Input: part model. Units: mm. Frame: model coordinates. A direction names the side the tool comes from. Coordinates: 2 decimals unless noted, no trailing zeros. Loops run counter-clockwise (first coordinate to the right, second up) from the corner with the lowest first, then second, coordinate; pieces in that order, holes last. Notation, with made-up numbers: (59.25, 34.5) -> (110.25, 34.5) arc R18 cw to (110.25, 43.5) -> close; hole circle Ø9 at (-7, 37). An arc over 180 degrees is marked (long way). Answer as a JSON object with one key per item and string values.
from build123d import *

# Parameters (mm, degrees)
SKETCH1_W            = 42
SKETCH1_H            = 84
SKETCH1_R            = 11.5
BOSS_EXTRUDE1_DEPTH  = 2
M3_CLEARANCE_HOLE1_D = 3.6
CHAMFER1_SIZE        = 4
BOSS_EXTRUDE2_DEPTH  = 42
CUT_EXTRUDE4_DEPTH   = 43


with BuildPart() as part:
    # Sketch1 → Boss-Extrude1 (new body)
    with BuildSketch(Plane.XY):
        with Locations((0, 21)):
            Rectangle(SKETCH1_W, SKETCH1_H)
        Circle(SKETCH1_R, mode=Mode.SUBTRACT)
    extrude(amount=BOSS_EXTRUDE1_DEPTH)

    # M3 Clearance Hole1 (through all)
    with Locations(Plane.XY.offset(2)):
        with Locations((-15.5, 15.5), (15.5, 15.5), (15.5, -15.5), (-15.5, -15.5)):
            Hole(M3_CLEARANCE_HOLE1_D / 2)

    # Chamfer1
    chamfer1_edges = [part.edges().sort_by_distance(p)[0] for p in [
        (-21, 63, 1),
        (21, 63, 1),
        (21, -21, 1),
        (-21, -21, 1),
    ]]
    chamfer(chamfer1_edges, length=CHAMFER1_SIZE)

    # Sketch4 → Boss-Extrude2 (add, through all)
    with BuildSketch(Plane(origin=(21, 0, 0), x_dir=(0, 0, -1), z_dir=(1, 0, 0))):
        Polygon((-32, 24), (-7.8, 59), (-2.8, 59), (-3.5, 24), (-2, 24), (-2, 19), (-32, 19), align=None)
    extrude(amount=-BOSS_EXTRUDE2_DEPTH)

    # Sketch5 → Cut-Extrude4 (cut, through all)
    with BuildSketch(Plane.ZY.offset(21)):
        Polygon((7.03069993, 22.5), (28.5, 22.5), (28.5, 22.907824173), (6.382789422, 54.895525423), align=None)
    extrude(amount=-CUT_EXTRUDE4_DEPTH, mode=Mode.SUBTRACT)


solid = part.part
1. Section query B-B (x = 0). Return loops of the section in (y, z).
Reply:
{"outline": "(-21, 0) -> (-11.5, 0) -> (-11.5, 2) -> (-21, 2) -> close; (11.5, 0) -> (63, 0) -> (63, 2) -> (24, 2) -> (24, 3.5) -> (59, 2.8) -> (59, 7.8) -> (24, 32) -> (19, 32) -> (19, 2) -> (11.5, 2) -> close; hole (22.5, 7.03) -> (54.9, 6.38) -> (22.91, 28.5) -> (22.5, 28.5) -> close"}
2. Pin query (flat end, axial travel): P1, Ø1, axis at x = 6.5, y = 35, coming from the +Z side; P2, Ø4, axis at x = 15.5, y = 15.5, coming from the +Z side; P3, Ø8, axis at x = 11, z = 23, coming from the -Y side. Return the tip coordinate at first contact, or that it passes through.
Reply:
{"P1": "stops at z = 24.74", "P2": "stops at z = 2", "P3": "stops at y = 19"}
3. Mould query, pull axis X, two halves, no side actions, for faces 1 (the face through (0, 24, 3)), 2 (the face through (21, 29, 6)), 3 (the face through (15.734, -13.715, 0.986)), 4 (the face through (15.734, 17.285, 0.986)). Classes: pulls with the +X half, pulls with the -X half, needs draft (parallel to the pull), parting line crosses it, or undercut.
Reply:
{"face 1": "needs draft", "face 2": "pulls with the +X half", "face 3": "undercut", "face 4": "undercut"}
4. Line query: line 1 along Y through (x, z) = (-15.5, 1.25); line 2 along Z through (x, y) = (-11, 54); line 3 along Z through (x, y) = (18.5, 42). Output: solid intervals per line, ascending.
Reply:
{"line 1": "y = -21 to -17.3, -13.7 to 13.7, 17.3 to 63", "line 2": "z = 0 to 2, 2.9 to 6.4, 7 to 11.26", "line 3": "z = 0 to 2, 3.14 to 6.64, 15.3 to 19.55"}
5. Section query C-C (y = -15.5). Return loops of the section in (x, z).
Reply:
{"outline": "(-21, 0) -> (-17.3, 0) -> (-17.3, 2) -> (-21, 2) -> close; (-13.7, 0) -> (13.7, 0) -> (13.7, 2) -> (-13.7, 2) -> close; (17.3, 0) -> (21, 0) -> (21, 2) -> (17.3, 2) -> close"}
6. Section query A-A (x = 15.5). Return loops of the section in (y, z), plus the area to 3 significant figures.
Reply:
{"outline": "(-21, 0) -> (-17.3, 0) -> (-17.3, 2) -> (-21, 2) -> close; (-13.7, 0) -> (13.7, 0) -> (13.7, 2) -> (-13.7, 2) -> close; (17.3, 0) -> (63, 0) -> (63, 2) -> (24, 2) -> (24, 3.5) -> (59, 2.8) -> (59, 7.8) -> (24, 32) -> (19, 32) -> (19, 2) -> (17.3, 2) -> close; hole (22.5, 7.03) -> (54.9, 6.38) -> (22.91, 28.5) -> (22.5, 28.5) -> close", "area": "538 mm2"}
7. Section query D-D (x = -12.5). Return loops of the section in (y, z), plus the area to 3 significant figures.
Reply:
{"outline": "(-21, 0) -> (63, 0) -> (63, 2) -> (24, 2) -> (24, 3.5) -> (59, 2.8) -> (59, 7.8) -> (24, 32) -> (19, 32) -> (19, 2) -> (-21, 2) -> close; hole (22.5, 7.03) -> (54.9, 6.38) -> (22.91, 28.5) -> (22.5, 28.5) -> close", "area": "552 mm2"}
8. Access query for faces 5 (the face through (-10, 8, 2)), 6 (the face through (0, 44, 2)), 7 (the face through (0, 22.5, 18)), 8 (the face through (-21, 29, 6)). Directions: +Z, -Z, +X, -X, +Y, -Y. A direction counts if a zero-diameter tool reaches every point of the face in a straight line with its end or side. Return the directions, or none.
Reply:
{"face 5": "+Z, +X, -X, -Y", "face 6": "+X, -X, +Y", "face 7": "+X, -X", "face 8": "+Z, -Z, -X, +Y, -Y"}
